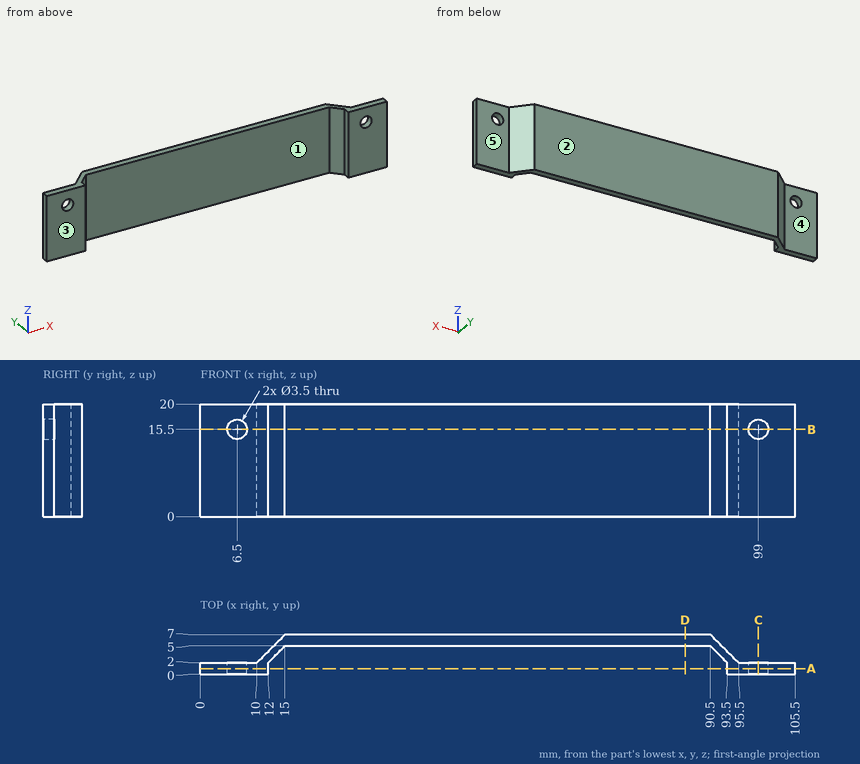
Study the drawing (mm; zero at the part's minimum x, y, z) and answer. A direction names the side the tool comes from. Coordinates: 2 decimals unless noted, no trailing zeros. Loops run counter-clockwise (first coordinate to the right, second up) from the corner with the lowest first, then second, coordinate; pieces in that order, holes last. Notation, with made-up numbers: (15.5, -19) -> (25.5, -19) arc R18 cw to (25.5, -9) -> close; hole circle Ø11 at (6, 66). An arc over 180 degrees is marked (long way). Answer as CSV lines item,"result".
1) The part is cut by section C-C (x = 99). Give the vertices of the cut face in (y, z), and give its area (3 significant figures).
A:
outline,"(0, 0) -> (2, 0) -> (2, 13.75) -> (0, 13.75) -> close; (0, 17.25) -> (2, 17.25) -> (2, 20) -> (0, 20) -> close"
area,"33.0 mm²"
2) The part is cut by section D-D (x = 86). Give the vertices of the cut face in (y, z), and give its area (3 significant figures).
A:
outline,"(5, 0) -> (7, 0) -> (7, 20) -> (5, 20) -> close"
area,"40.0 mm²"
3) For the marked faces 1, 2, 3, 4 and 5, determine the directions among +Z, -Z, +X, -X, +Y, -Y from which every point of the face is accessible in a straight line to the end or side of a thin tool.
A:
face 1,"+Z, -Z, -Y"
face 2,"+Z, -Z, +X, -X, +Y"
face 3,"+Z, -Z, +X, -X, -Y"
face 4,"+Z, -Z, -X, +Y"
face 5,"+Z, -Z, +X, +Y"
4) Flat-ended cylindrical pins translate along their axes: pin 1 (5 mm diameter, centred on x = 18, z = 16.5, fed in from -Y); pin 2 (1 mm diameter, centred on y = 4.5, z = 17, fed in from +X); pin 3 (4 mm diameter, centred on y = 5.5, z = 4, fed in from -X). Find the tip coordinate at first contact, or state that the pin passes through.
A:
pin 1,"stops at y = 5"
pin 2,"stops at x = 93.5"
pin 3,"stops at x = 11.5"
5) The part is cut by section A-A (y = 1). Give the vertices of the cut face in (x, z).
A:
outline,"(0, 0) -> (12, 0) -> (12, 20) -> (0, 20) -> close; (93.5, 0) -> (105.5, 0) -> (105.5, 20) -> (93.5, 20) -> close; hole circle Ø3.5 at (6.5, 15.5); hole circle Ø3.5 at (99, 15.5)"
6) Straight lines are drawn through the part: probe 1 along X at (y, z) = (1, 15.5); probe 2 along X at (y, z) = (1.25, 3); probe 3 along Z at (x, y) = (99, 1.15). For each, find the intervals that lie inside material, in ascending order.
A:
probe 1,"x = 0 to 4.75, 8.25 to 12, 93.5 to 97.25, 100.75 to 105.5"
probe 2,"x = 0 to 12, 93.5 to 105.5"
probe 3,"z = 0 to 13.75, 17.25 to 20"
7) The part is cut by section B-B (z = 15.5). Give the vertices of the cut face in (x, y).
A:
outline,"(0, 0) -> (4.75, 0) -> (4.75, 2) -> (0, 2) -> close; (8.25, 0) -> (12, 0) -> (12, 2) -> (15, 5) -> (90.5, 5) -> (93.5, 2) -> (93.5, 0) -> (97.25, 0) -> (97.25, 2) -> (95.5, 2) -> (90.5, 7) -> (15, 7) -> (10, 2) -> (8.25, 2) -> close; (100.75, 0) -> (105.5, 0) -> (105.5, 2) -> (100.75, 2) -> close"
